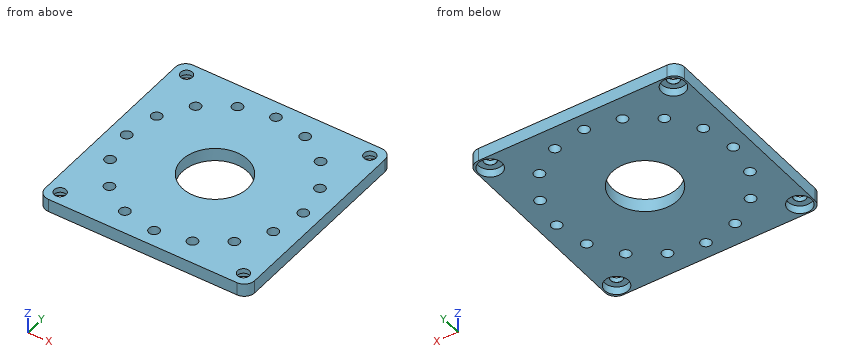
```python
from build123d import *

# Parameters (mm, degrees)
ESQUISSE1_R                                = 12.5
ESQUISSE1_R_2                              = 2
BOSS_EXTRU_1_DEPTH                         = 5
D_GAGEMENT_M41_D                           = 4.5
CHAMBRAGE_POUR_VIS_T_TE_RONDE_BOMB_2_COUNT = 2
CHAMBRAGE_POUR_VIS_T_TE_RONDE_BOMB_2_PITCH = 69.975976343
CHAMBRAGE_POUR_VIS_T_TE_RONDE_BOMB_3_COUNT = 2
CHAMBRAGE_POUR_VIS_T_TE_RONDE_BOMB_3_PITCH = 98.968247754
CHAMBRAGE_POUR_VIS_T_TE_RONDE_BOMB_4_COUNT = 2
CHAMBRAGE_POUR_VIS_T_TE_RONDE_BOMB_4_PITCH = 69.986261497


with BuildPart() as part:
    # Esquisse1 → Boss.-Extru.1 (new body)
    with BuildSketch(Plane.XY):
        with BuildLine():
            Line((-36, -40), (36, -40))
            ThreePointArc((36, -40), (38.828427125, -38.828427125), (40, -36))
            Line((40, -36), (40, 36))
            ThreePointArc((40, 36), (38.828427125, 38.828427125), (36, 40))
            Line((36, 40), (-36, 40))
            ThreePointArc((-36, 40), (-38.828427125, 38.828427125), (-40, 36))
            Line((-40, 36), (-40, -36))
            ThreePointArc((-40, -36), (-38.828427125, -38.828427125), (-36, -40))
        make_face()
        Circle(ESQUISSE1_R, mode=Mode.SUBTRACT)
        with Locations((0, 33.738776676)):
            Circle(ESQUISSE1_R_2, mode=Mode.SUBTRACT)
        with Locations((12.911270862, 31.170565223)):
            Circle(ESQUISSE1_R_2, mode=Mode.SUBTRACT)
        with Locations((23.856917777, 23.856917777)):
            Circle(ESQUISSE1_R_2, mode=Mode.SUBTRACT)
        with Locations((31.170565223, 12.911270862)):
            Circle(ESQUISSE1_R_2, mode=Mode.SUBTRACT)
        with Locations((33.738776676, 0)):
            Circle(ESQUISSE1_R_2, mode=Mode.SUBTRACT)
        with Locations((31.170565223, -12.911270862)):
            Circle(ESQUISSE1_R_2, mode=Mode.SUBTRACT)
        with Locations((23.856917777, -23.856917777)):
            Circle(ESQUISSE1_R_2, mode=Mode.SUBTRACT)
        with Locations((12.911270862, -31.170565223)):
            Circle(ESQUISSE1_R_2, mode=Mode.SUBTRACT)
        with Locations((0, -33.738776676)):
            Circle(ESQUISSE1_R_2, mode=Mode.SUBTRACT)
        with Locations((-12.911270862, -31.170565223)):
            Circle(ESQUISSE1_R_2, mode=Mode.SUBTRACT)
        with Locations((-23.856917777, -23.856917777)):
            Circle(ESQUISSE1_R_2, mode=Mode.SUBTRACT)
        with Locations((-31.170565223, -12.911270862)):
            Circle(ESQUISSE1_R_2, mode=Mode.SUBTRACT)
        with Locations((-33.738776676, 0)):
            Circle(ESQUISSE1_R_2, mode=Mode.SUBTRACT)
        with Locations((-31.170565223, 12.911270862)):
            Circle(ESQUISSE1_R_2, mode=Mode.SUBTRACT)
        with Locations((-23.856917777, 23.856917777)):
            Circle(ESQUISSE1_R_2, mode=Mode.SUBTRACT)
        with Locations((-12.911270862, 31.170565223)):
            Circle(ESQUISSE1_R_2, mode=Mode.SUBTRACT)
    extrude(amount=BOSS_EXTRU_1_DEPTH)

    # Dégagement M41 (through all)
    with Locations(Plane.XY.offset(5)):
        with Locations((-34.968353645, 34.962380164), (-34.968353645, -35.023881333), (35.007622699, -35.023881333), (35.007622699, 34.962380164)):
            Hole(D_GAGEMENT_M41_D / 2)

    # Esquisse10 → Chambrage pour vis à tête ronde bombée M41 (revolve, cut)
    with BuildSketch(Plane(origin=(35.007622699, 34.962380164, 0), x_dir=(0, 1, 0), z_dir=(1, 0, 0))):
        Polygon((0, 0), (0, 5), (2.25, 5), (2.25, 3.125), (2.275, 3.1), (4.5, 3.1), (4.5, 0), align=None)
    chambrage_pour_vis_t_te_ronde_bomb_e_m = revolve(axis=Axis((35.007622699, 34.962380164, -6.35), (0, 0, 1)), mode=Mode.SUBTRACT)

    # Chambrage pour vis _ t_te ronde bomb 2: Chambrage pour vis à tête ronde bombée M41 ×2
    with Locations(*[(-i * CHAMBRAGE_POUR_VIS_T_TE_RONDE_BOMB_2_PITCH, 0, 0) for i in range(1, CHAMBRAGE_POUR_VIS_T_TE_RONDE_BOMB_2_COUNT)]):
        add(chambrage_pour_vis_t_te_ronde_bomb_e_m, mode=Mode.SUBTRACT)

    # Chambrage pour vis _ t_te ronde bomb 3: Chambrage pour vis à tête ronde bombée M41 ×2
    with Locations(*[Vector(-0.7070548173920428, -0.7071587411626226, 0) * (i * CHAMBRAGE_POUR_VIS_T_TE_RONDE_BOMB_3_PITCH) for i in range(1, CHAMBRAGE_POUR_VIS_T_TE_RONDE_BOMB_3_COUNT)]):
        add(chambrage_pour_vis_t_te_ronde_bomb_e_m, mode=Mode.SUBTRACT)

    # Chambrage pour vis _ t_te ronde bomb 4: Chambrage pour vis à tête ronde bombée M41 ×2
    with Locations(*[(0, -i * CHAMBRAGE_POUR_VIS_T_TE_RONDE_BOMB_4_PITCH, 0) for i in range(1, CHAMBRAGE_POUR_VIS_T_TE_RONDE_BOMB_4_COUNT)]):
        add(chambrage_pour_vis_t_te_ronde_bomb_e_m, mode=Mode.SUBTRACT)


solid = part.part
```
Model file for the job. Use its own axes, mm. Give positions to 0.01 mm unless a question says otherwise; leave off trailing zeros. Loops run counter-clockwise (first coordinate to the right, second up) from the corner with the lowest first, then second, coordinate; pieces in that order, holes last. Notation, with made-up numbers: M 17.5,80.5 L 53.5,80.5 A30 ccw 53.5,112.5 Z; hole C -20.75,76.25 d2. An arc over 180 degrees is marked long. Use one line per item in the form item = value.
Item 1: Slice it at C-C on z = 1.1. Give the number of separate pieces and of enclosed holes in the cut face, and give its area (3 significant figures).
Filled in:
separate_pieces = 1
enclosed_holes = 21
area = 5,440 mm^2
Item 2: Drill centre lines: L1, parallel to X at y = -25, z = 3.45; L2, parallel to X at y = 1.5, z = 1.35; L3, parallel to Y at x = -33.5, z = 1.9. Where is each one in solid material? Low to high.
Filled in:
L1 = -40 to -25.5, -22.22 to 22.22, 25.5 to 40
L2 = -40 to -35.06, -32.42 to -12.41, 12.41 to 32.42, 35.06 to 40
L3 = -40 to -39.28, -30.77 to -1.99, 1.99 to 30.71, 39.22 to 40
Item 3: Slice it at A-A on y = 0. List the corners of the cut face in (x, z).
Filled in:
outline = M -40,0 L -35.74,0 L -35.74,5 L -40,5 Z; M -31.74,0 L -12.5,0 L -12.5,5 L -31.74,5 Z; M 12.5,0 L 31.74,0 L 31.74,5 L 12.5,5 Z; M 35.74,0 L 40,0 L 40,5 L 35.74,5 Z
Item 4: Flat gauge pin, fed straight in: pin 1 Ø5 at (x, y) = (-34.97, 34.96) entering from -Z. Where does the tip first touch, or does it go through?
Filled in:
pin_1 = 3.1
Item 5: Slice it at D-D on y = 8. List the corners of the cut face in (x, z).
Filled in:
outline = M -40,0 L -9.6,0 L -9.6,5 L -40,5 Z; M 9.6,0 L 40,0 L 40,5 L 9.6,5 Z
